The figure shows three views and two pictorial views of one solid part (mm, origin at its lowest corner). Answer the questions. A direction names the side the tool comes from. Round coordinates to 2 decimals unless told otherwise and drop trailing zeros. Order: outer loops, then holes, each group sorted by start corner. A loop starts at its lowest first (then second) coordinate and runs counter-clockwise, first axis right, second up. Notation, with made-up numbers: (85.5, 86.25) - (90.5, 86.25) arc R22 cw to (90.5, 112.25) - close; hole circle Ø7 at (38.5, 41.5). An arc over 180 degrees is marked (long way). Use CSV: the item, a comma, the result in double quotes.
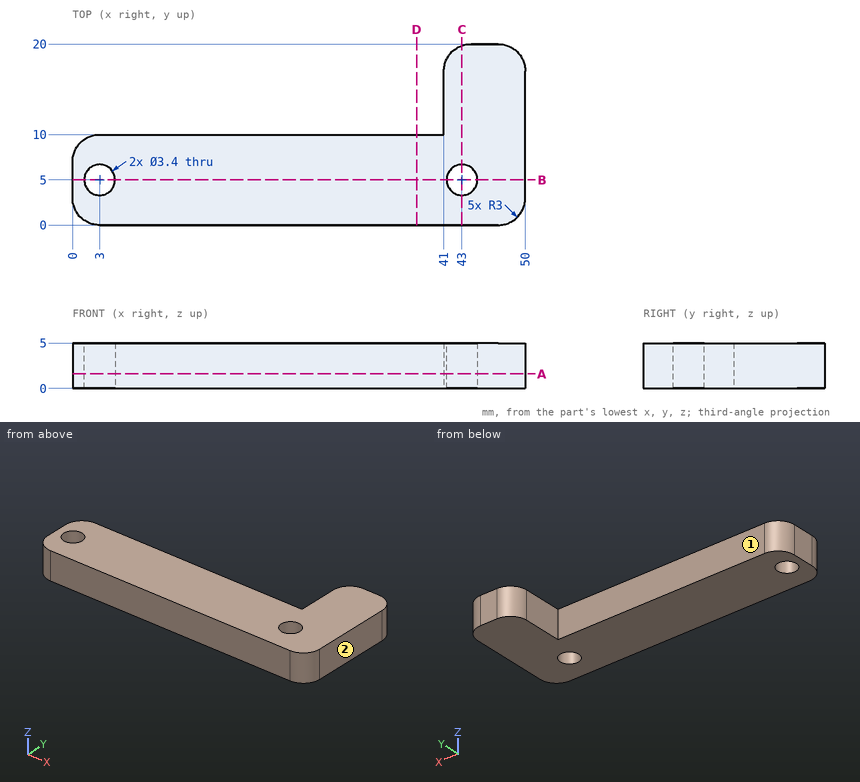
(1) For the marked faces 1 and 2, determine the directions among +Z, -Z, +X, -X, +Y, -Y from which every point of the face is accessible in a straight line to the end or side of a thin tool.
Findings below:
face 1,"+Z, -Z, -X, +Y"
face 2,"+Z, -Z, +X, +Y, -Y"
(2) Find section C-C (x = 43). Determine the outline of the cut face in (y, z), and give its area (3 significant figures).
Findings below:
outline,"(0, 0) - (3.3, 0) - (3.3, 5) - (0, 5) - close; (6.7, 0) - (19.83, 0) - (19.83, 5) - (6.7, 5) - close"
area,"82.1 mm²"
(3) Each of these flat-tipped pins is pushed along its axis until it touches: pin 1 (1.5 mm diameter, centred on y = 12.5, z = 1.5, fed in from -X); pin 2 (2 mm diameter, centred on x = 17.5, y = 8.5, fed in from -Z); pin 3 (2.5 mm diameter, centred on x = 16.5, z = 1.5, fed in from +Y). Where does it stop, or does it pass through?
Findings below:
pin 1,"stops at x = 41"
pin 2,"stops at z = 0"
pin 3,"stops at y = 10"
(4) Find section B-B (y = 5). Determine the outline of the cut face in (x, z).
Findings below:
outline,"(0, 0) - (1.3, 0) - (1.3, 5) - (0, 5) - close; (4.7, 0) - (41.3, 0) - (41.3, 5) - (4.7, 5) - close; (44.7, 0) - (50, 0) - (50, 5) - (44.7, 5) - close"
(5) Find section D-D (x = 38). Determine the outline of the cut face in (y, z), and give its area (3 significant figures).
Findings below:
outline,"(0, 0) - (10, 0) - (10, 5) - (0, 5) - close"
area,"50.0 mm²"
(6) Find section A-A (z = 1.6). Determine the outline of the cut face in (x, y), and give its area (3 significant figures).
Findings below:
outline,"(0, 3) arc R3 ccw to (3, 0) - (47, 0) arc R3 ccw to (50, 3) - (50, 17) arc R3 ccw to (47, 20) - (44, 20) arc R3 ccw to (41, 17) - (41, 10) - (3, 10) arc R3 ccw to (0, 7) - close; hole circle Ø3.4 at (3, 5); hole circle Ø3.4 at (43, 5)"
area,"562 mm²"
(7) Find the intervals of material crossed by L1, parallel to Y at x = 3, z = 3.6; L2, parallel to X at y = 14, z = 0.9; L3, parallel to Y at x = 23, z = 2.65, in increasing order. Write a range as from..to.
Findings below:
L1,"y = 0..3.3, 6.7..10"
L2,"x = 41..50"
L3,"y = 0..10"
